Read the model definition and answer for the solid it produces. Units are mm, in the model's axes. Face numbers are marked on the shaded views. Coordinates: 2 decimals unless noted, no trailing zeros. Loops run counter-clockwise (first coordinate to the right, second up) from the corner with the lowest first, then second, coordinate; pieces in that order, holes last. Notation, with made-up numbers: (39, 83.5) -> (45, 83.5) arc R24 cw to (45, 99.5) -> close; hole circle Ø9 at (8.5, -34.5). An arc over 180 degrees is marked (long way). Answer as a JSON object with one key per item and string values. Group by question number.
Q1. Straight lines are drawn through the part: line 1 along Y through (x, z) = (5, 0) (3 decimals); line 2 along Y through (x, z) = (-0.75, 2.25); line 3 along X through (y, z) = (14, 0.25). For each, find the intervals that lie inside material, in ascending order. Write a range as [from, to].
Q2. Each of these flat-tipped pins is pushed along its axis until it touches: P1, Ø2.5, axis at x = 0.5, z = 0.5, coming from the -Y side; P2, Ø6, axis at y = 20, z = 3.5, coming from the +X side. Where does it stop, or does it pass through?
Q3. The part is cut by section D-D on z = -2.25. Write down the section's boundary in (x, y).
Q4. The part is cut by section A-A on z = 0. Write down the section's boundary in (x, y) (3 decimals), and give its area (3 significant figures).
Q5. The part is cut by section C-C on y = 18. Write down the section's boundary in (x, z) (3 decimals), and give its area (3 significant figures).
Q6. The part is cut by section B-B on x = 0. Write down the section's boundary in (y, z) (3 decimals).
Q7. Determine the mould class of the marked faces 1, 2 and 3 for opening direction X: released by +X, released by -X, zero draft, split by the parting line, or undercut.
from build123d import *

# Parameters (mm, degrees)
BOSS_EXTRUDE1_DEPTH      = 57.15
BOSS_EXTRUDE2_DEPTH      = 57.15
BOSS_EXTRUDE3_START      = -6.35
BOSS_EXTRUDE3_DEPTH      = 6.35
SKETCH5_R                = 3.96875
CUT_EXTRUDE1_DEPTH       = 6.35
BOSS_EXTRUDE4_DEPTH      = 6.35
BOSS_EXTRUDE4_DEPTH_BACK = 33.147
SKETCH7_R                = 5.715
SKETCH7_R_2              = 3.96875
CUT_EXTRUDE2_DEPTH       = 59.440702853
CUT_EXTRUDE2_DEPTH_BACK  = 59.440702853
SKETCH6_R                = 1.75


with BuildPart() as part:
    # Sketch1 → Boss-Extrude1 (new body)
    with BuildSketch(Plane(origin=(0, 0, 0), x_dir=(1, 0, 0), z_dir=(0, 1, 0))):
        with BuildLine():
            Line((-4.099560952, 3), (4.099560952, 3))
            ThreePointArc((4.099560952, 3), (0, -5.08), (-4.099560952, 3))
        make_face()
    extrude(amount=BOSS_EXTRUDE1_DEPTH)

    # Sketch3 → Boss-Extrude2 (add)
    with BuildSketch(Plane.XZ):
        with BuildLine():
            Line((-4.099560952, -3), (4.099560952, -3))
            ThreePointArc((4.099560952, -3), (0, -5.08), (-4.099560952, -3))
        make_face()
    extrude(amount=-BOSS_EXTRUDE2_DEPTH)

    # Sketch4 → Boss-Extrude3 (add)
    with BuildSketch(Plane(origin=(0, 57.15, 0), x_dir=(1, 0, 0), z_dir=(0, 1, 0)).offset(BOSS_EXTRUDE3_START)):
        with BuildLine():
            Line((-4.099560952, 3), (4.099560952, 3))
            ThreePointArc((4.099560952, 3), (0, 5.08), (-4.099560952, 3))
        make_face()
    extrude(amount=BOSS_EXTRUDE3_DEPTH)

    # Sketch5 → Cut-Extrude1 (cut)
    with BuildSketch(Plane.XZ):
        with Locations(Location((0, 0, 0), (0, 0, 270))):
            Circle(SKETCH5_R)
    extrude(amount=-CUT_EXTRUDE1_DEPTH, mode=Mode.SUBTRACT)

    # Sketch7 → Boss-Extrude4 (add, two sides: drawn at the far end of the back side and taken through both)
    with BuildSketch(Plane(origin=(0, 6.35, 0), x_dir=(-1, 0, 0), z_dir=(0, -1, 0)).offset(-BOSS_EXTRUDE4_DEPTH_BACK)):
        with Locations(Location((0, 0, 0), (0, 0, 90))):
            Circle(SKETCH7_R)
        with Locations(Location((0, 0, 0), (0, 0, 90))):
            Circle(SKETCH7_R_2, mode=Mode.SUBTRACT)
    extrude(amount=BOSS_EXTRUDE4_DEPTH + BOSS_EXTRUDE4_DEPTH_BACK)

    # Sketch6 → Cut-Extrude2 (cut, two sides: drawn at the far end of the back side and taken through both)
    with BuildSketch(Plane(origin=(5.08, 0, 0), x_dir=(0, 0, -1), z_dir=(1, 0, 0)).offset(-CUT_EXTRUDE2_DEPTH_BACK)):
        with Locations((0, 3.175)):
            Circle(SKETCH6_R)
    extrude(amount=CUT_EXTRUDE2_DEPTH + CUT_EXTRUDE2_DEPTH_BACK, mode=Mode.SUBTRACT)


solid = part.part
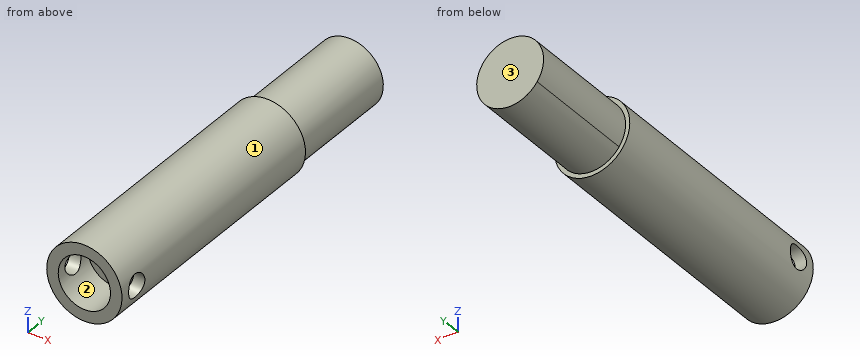
Final values:
{
 "1": {"line 1": "y = [0, 1.425], [4.925, 57.15]", "line 2": "y = [6.35, 57.15]", "line 3": "x = [-5.71, 5.71]"},
 "2": {"P1": "stops at y = 6.35", "P2": "stops at x = 5.69"},
 "3": {"outline": "(-5.25, 0) -> (-3.27, 0) -> (-3.27, 6.35) -> (3.27, 6.35) -> (3.27, 0) -> (5.25, 0) -> (5.25, 39.5) -> (4.55, 39.5) -> (4.55, 57.15) -> (-4.55, 57.15) -> (-4.55, 39.5) -> (-5.25, 39.5) -> close"},
 "4": {"outline": "(-5.715, 0) -> (-3.969, 0) -> (-3.969, 1.425) -> (-5.715, 1.425) -> close; (-5.715, 4.925) -> (-3.969, 4.925) -> (-3.969, 6.35) -> (3.969, 6.35) -> (3.969, 4.925) -> (5.715, 4.925) -> (5.715, 39.497) -> (5.08, 39.497) -> (5.08, 57.15) -> (-5.08, 57.15) -> (-5.08, 39.497) -> (-5.715, 39.497) -> close; (3.969, 0) -> (5.715, 0) -> (5.715, 1.425) -> (3.969, 1.425) -> close", "area": "568 mm2"},
 "5": {"outline": "circle Ø11.43 at (0, 0)", "area": "103 mm2"},
 "6": {"outline": "(0, -5.715) -> (39.497, -5.715) -> (39.497, -5.08) -> (57.15, -5.08) -> (57.15, 5.08) -> (39.497, 5.08) -> (39.497, 5.715) -> (0, 5.715) -> (0, 3.969) -> (6.35, 3.969) -> (6.35, -3.969) -> (0, -3.969) -> close"},
 "7": {"face 1": "split by the parting line", "face 2": "undercut", "face 3": "zero draft"}
}
